Geometry: final body of the model. Coordinates: model frame, mm. A direction names the side the tool comes from. Round coordinates to 2 decimals unless told otherwise and drop trailing zeros. Loops run counter-clockwise (first coordinate to the right, second up) from the corner with the lowest first, then second, coordinate; pieces in that order, holes last. Notation, with made-up numbers: M 36.25,7 L 59.25,7 A27 ccw 59.25,34 Z; hole C 29.5,71 d7. An arc over 180 degrees is marked long. Return JSON: item names as keys, results as strings.
Autodesk Inventor part; units mm, degrees
ref_plane "YZ Plane" through (0, 0, 0) normal (1, 0, 0) x (0, 1, 0)
ref_plane "XZ Plane" through (0, 0, 0) normal (0, 1, 0) x (-1, 0, 0)
ref_plane "XY Plane" through (0, 0, 0) normal (0, 0, 1) x (1, 0, 0)
sketch "Sketch1" plane through (0, 0, 0) normal (0, 0, 1) x (1, 0, 0)
  line L0 (0, 0) -> (0, 16) construction
  line L1 (0, 16) -> (2.5, 16) construction
  line L2 (2.5, 16) -> (9, 16)
  line L3 (9, 16) -> (9, 15)
  line L4 (9, 15) -> (6.1, 15)
  line L5 (6.1, 15) -> (6.1, 7.5)
  line L6 (6.1, 7.5) -> (9, 7.5)
  line L7 (9, 7.5) -> (9, 0)
  line L8 (9, 0) -> (2.5, 0)
  line L9 (2.5, 0) -> (2.5, 16)
  dimension "d0" = 2.5
  dimension "d1" = 7.5
  dimension "d2" = 7.5
  dimension "d3" = 9
  dimension "d4" = 1
  dimension "d6" = 6.1
revolve "Revolution1" add sketch "Sketch1" angle 360 about axis through (0, 0, 0) along (0, 1, 0)
sketch "Sketch2" plane through (0, 7.5, 0) normal (0, 1, 0) x (1, 0, 0)
  line L0 (0, 0) -> (0, -6.7)
  circle A0 centre (0, -6.7) radius 1
  dimension "d8" = 2
  dimension "d9" = 6.7
extrude "Extrusion1" cut sketch "Sketch2" along normal up to surface (7.5 mm away)
pattern_circular "Circular Pattern1" count 20 over 360 about axis through (0, 11.25, 0) along (0, -1, 0) of "Extrusion1"
properties part number "gt2 20t pulley"
Q1. Section query A-A (x = 0). Output: boundary loops of the cut face in (y, z).
Determined:
{"outline": "M 0,-9 L 7.5,-9 L 7.5,-5.7 L 15,-5.7 L 15,-9 L 16,-9 L 16,-2.5 L 0,-2.5 Z; M 0,2.5 L 16,2.5 L 16,9 L 15,9 L 15,5.7 L 7.5,5.7 L 7.5,9 L 0,9 Z"}
Q2. Material intervals for L1, parallel to Z at x = 0, y = 12.75; L2, parallel to Z at x = 0, y = 6.25; L3, parallel to Y at x = 0.25, z = 7.25, sorted ascending.
Determined:
{"L1": "z = -5.7 to -2.5, 2.5 to 5.7", "L2": "z = -9 to -2.5, 2.5 to 9", "L3": "y = 0 to 7.5, 15 to 16"}
Q3. Pull-direction query (Y, two-part tool) for faces 1 (the flat face through (2, 0, 2)), 2 (the flat face through (2, 16, 2)), 3 (the cylindrical face through (5.425, 11.198, -1.75)); classes: pulls with the +Y half, pulls with the -Y half, needs draft (parallel to the pull), parting line crosses it, or undercut.
Determined:
{"face 1": "pulls with the -Y half", "face 2": "pulls with the +Y half", "face 3": "undercut"}
Q4. Section query C-C (z = -5). Output: boundary loops of the cut face in (x, y).
Determined:
{"outline": "M -7.48,0 L 7.48,0 L 7.48,7.5 L 3.03,7.5 L 3.03,15 L 7.48,15 L 7.48,16 L -7.48,16 L -7.48,15 L -3.03,15 L -3.03,7.5 L -7.48,7.5 Z"}
Q5. Pin query (flat end, axial travel): pin 1 (5 mm diameter, centred on y = 6, z = 5.5, fed in from -X); pin 2 (5 mm diameter, centred on y = 3, z = -6, fed in from +X); pin 3 (4.5 mm diameter, centred on x = 0, z = 0, fed in from +Y); pin 4 (8 mm diameter, centred on y = 6, z = 6.5, fed in from -X). Return the tip coordinate at first contact, or that it passes through.
Determined:
{"pin 1": "stops at x = -8.49", "pin 2": "stops at x = 8.29", "pin 3": "passes through", "pin 4": "stops at x = -8.65"}
Q6. Section query D-D (y = 2). Output: boundary loops of the cut face in (x, z), plus the area to 3 significant figures.
Determined:
{"outline": "C 0,0 d18; hole C 0,0 d5", "area": "235 mm^2"}
Q7. Reachability of faces 4 (the flat face through (0, 15, 6)), 5 (the cylindrical face through (-3.34, 11.2, -4.62)), 6 (the cylindrical face through (-1.77, 11.2, 5.42)) from +Z, -Z, +X, -X, +Y, -Y: full face, straight path, thin tool, end or side. Return the list, or none.
Determined:
{"face 4": "none", "face 5": "-Z", "face 6": "+Z"}
Q8. Section query B-B (z = 0). Output: boundary loops of the cut face in (x, y).
Determined:
{"outline": "M -9,0 L -2.5,0 L -2.5,16 L -9,16 L -9,15 L -5.7,15 L -5.7,7.5 L -9,7.5 Z; M 2.5,0 L 9,0 L 9,7.5 L 5.7,7.5 L 5.7,15 L 9,15 L 9,16 L 2.5,16 Z"}
